Verification items for the finished model (mm, model axes). Round coordinates to 2 decimals unless told otherwise and drop trailing zeros. Write each loop counter-clockwise with the first axis right and the second up, starting at its lowest first coordinate (ties: lowest second). Pieces come first, ordered by that corner, then holes. Notation, with made-up numbers: (27, 14.25) -> (70, 14.25) arc R32 cw to (70, 44.25) -> close; hole circle Ø10 at (79.5, 14.25). An arc over 180 degrees is marked (long way). Answer as a JSON object with one key per item and string values. Group by question number.
(1) Draft check along X on faces 1 (the face through (-1, 50.8, 31)), 2 (the face through (49.272, -0.64, -49.351)), 3 (the face through (24.227, -0.637, 7.629)). Enter one of: released by +X, released by -X, zero draft, split by the parting line, or undercut.
(2) Sectioned sample at A-A on y = 27. Record the cut outline in (x, z), and give its area (3 significant figures).
(3) Scan lines: L1, parallel to Z at x = 0, y = 12; L2, parallel to X at y = -31.5, z = 1; L3, parallel to Z at x = -17.5, y = 43.5. Record each from-to range of solid material in increasing order. Write a range as from..to.
```python
from build123d import *

# Parameters (mm, degrees)
F0_W     = 101.6
F0_H     = 101.6
F1_DEPTH = 50.8
F2_R     = 25.4
F3_DEPTH = 101.601
F4_SIZE  = 3.175
F5_R     = 5.08


with BuildPart() as f1:
    # F0 (on Front) → F1 (new body, symmetric)
    with BuildSketch(Plane.XZ):
        Rectangle(F0_W, F0_H)
    extrude(amount=F1_DEPTH, both=True)

    # F2 (on face) → F3 (cut, through all)
    with BuildSketch(Plane.XZ.offset(50.8)):
        Circle(F2_R)
    extrude(amount=-F3_DEPTH, mode=Mode.SUBTRACT)

    # F4
    f4_edges = [f1.edges().sort_by_distance(p)[0] for p in [
        (-25.4, -50.8, 0),
        (-25.4, 50.8, 0),
    ]]
    chamfer(f4_edges, length=F4_SIZE)

    # F5
    f5_edges = [f1.edges().sort_by_distance(p)[0] for p in [
        (50.8, 0, -50.8),
        (50.8, 0, 50.8),
        (0, 50.8, 50.8),
        (-50.8, 0, 50.8),
        (0, -50.8, 50.8),
        (-50.8, 0, -50.8),
        (0, 50.8, -50.8),
        (0, -50.8, -50.8),
        (-50.8, 50.8, 0),
        (-50.8, -50.8, 0),
        (50.8, 50.8, 0),
        (50.8, -50.8, 0),
        (26.9875, 49.2125, 0),
        (-28.575, 50.8, 0),
        (-25.4, 47.625, 0),
        (25.4, 0, 0),
        (-25.4, -47.625, 0),
        (26.9875, -49.2125, 0),
        (-28.575, -50.8, 0),
    ]]
    fillet(f5_edges, radius=F5_R)


solid = f1.part
```
Computed values:
{
 "1": {"face 1": "zero draft", "face 2": "released by +X", "face 3": "undercut"},
 "2": {"outline": "(-50.8, -45.72) arc R5.08 ccw to (-45.72, -50.8) -> (45.72, -50.8) arc R5.08 ccw to (50.8, -45.72) -> (50.8, 45.72) arc R5.08 ccw to (45.72, 50.8) -> (-45.72, 50.8) arc R5.08 ccw to (-50.8, 45.72) -> close; hole circle Ø50.8 at (0, 0)", "area": "8,270 mm2"},
 "3": {"L1": "-50.8..-25.4, 25.4..50.8", "L2": "-50.8..-25.38, 25.38..50.8", "L3": "-50.8..-18.41, 18.41..50.8"}
}
